Autodesk Inventor part; units mm, degrees
ref_plane "Work Plane1" through (0, 5, -20) normal (0, 1, 0) x (1, 0, 0)
ref_plane "YZ Plane" through (0, 0, 0) normal (1, 0, 0) x (0, 1, 0)
ref_plane "XZ Plane" through (0, 0, 0) normal (0, 1, 0) x (-1, 0, 0)
sketch "Sketch1" plane through (0, 0, 0) normal (1, 0, 0) x (0, 1, 0)
  line L0 (0, 0) -> (5, 0)
  line L1 (5, 0) -> (5, -40)
  line L2 (5, -40) -> (0, -40)
  line L3 (0, -40) -> (0, 0)
  line L4 (0, 0) -> (2.5, 0)
  line L5 (2.5, 0) -> (2.5, 16)
  line L6 (2.5, 16) -> (0, 16)
  line L7 (0, 16) -> (0, 0)
  line L8 (0, -40) -> (2.5, -40)
  line L9 (2.5, -40) -> (2.5, -54)
  line L10 (2.5, -54) -> (0, -54)
  line L11 (0, -54) -> (0, -40)
  line L12 (0, -54) -> (2.5, -54)
  line L13 (2.5, -54) -> (2.5, -61.5)
  line L14 (2.5, -61.5) -> (0, -61.5)
  line L15 (0, -61.5) -> (0, -54)
  line L16 (0, 16) -> (2, 16)
  line L17 (0, 14) -> (0, 16)
  line L18 (0, 19.99) -> (0, -68.5807)
  point P0 (2.5, -40)
  dimension "d0" = 5
  dimension "d1" = 40
  dimension "d2" = 2.5
  dimension "d3" = 16
  dimension "d4" = 2.5
  dimension "d5" = 14
  dimension "d6" = 2.5
  dimension "d7" = 7.5
revolve "Revolution1" add sketch "Sketch1" angle 360 about axis through (0, 0, 19.99) along (0, 0, -1)
sketch "Sketch4" plane through (0, 0, 0) normal (0, 0, 1) x (1, 0, 0)
  circle A0 centre (0, 0) radius 5 construction
  line L0 (0, 5) -> (2.5, 5)
  line L1 (2.5, 5) -> (-2.5, 5)
  line L2 (-2.5, 5) -> (-2.5, 3.5)
  line L3 (-2.5, 3.5) -> (2.5, 3.5)
  line L4 (2.5, 3.5) -> (2.5, 5)
  point P0 (0, 0)
  dimension "d25" = 2.5
  dimension "d26" = 5
  dimension "d27" = 1.5
extrude "Extrusion3" cut sketch "Sketch4" against normal blind 5.5
sketch "Sketch5" plane through (0, 0, -40) normal (0, 0, -1) x (-1, 0, 0)
  circle A0 centre (0, 0) radius 5 construction
  line L0 (0, 5) -> (2.5, 5)
  line L1 (-2.5, 4.3301) -> (-2.5, 3.5)
  line L2 (2.5, 5) -> (-2.5, 5)
  line L3 (-2.5, 5) -> (-2.5, 3.5)
  line L4 (-2.5, 3.5) -> (2.5, 3.5)
  line L5 (2.5, 3.5) -> (2.5, 5)
  point P0 (0, 0)
  dimension "d30" = 2.5
  dimension "d31" = 5
  dimension "d32" = 1.5
extrude "Extrusion4" cut sketch "Sketch5" against normal blind 5.5
ref_plane "Work Plane1" through (0, 5, -20) normal (0, 1, 0) x (1, 0, 0)
sketch "Sketch6" plane through (0, 5, -20) normal (0, 1, 0) x (1, 0, 0)
  line L0 (2.5, -14.5) -> (-2.5, -14.5)
  circle A0 centre (0, -14.5) radius 2.5
  line L1 (-2.5, 14.5) -> (2.5, 14.5)
  circle A1 centre (0, 14.5) radius 2.5
  point P0 (0, -20)
extrude "Extrusion5" cut sketch "Sketch6" against normal blind 1.5
fillet "Fillet2" radius 0.5 2 edges at (0, -2.5, 0) (0, -2.5, -40)
fillet "Fillet3" radius 0.25 6 edges at (0, 3.5, -8) (2.5, 3.5, -2.75) (-2.5, 3.5, -2.75) (0, 3.5, -32) (2.5, 3.5, -37.25) (-2.5, 3.5, -37.25)
properties part number "eje2" material "PBT Plastic"
Can you work these out from the model? Positions are in its coordinate system, mm. A direction names the side the tool comes from. Round coordinates to 2 decimals unless told otherwise and drop trailing zeros. Order: outer loops, then holes, each group sorted by start corner. A loop starts at its lowest first (then second) coordinate and runs counter-clockwise, first axis right, second up.
(1) If I drill on L1, parallel to Z at x = -3, y = 2.5; L2, parallel to Y at x = -0.5, z = -7.5; L3, parallel to X at y = 0.75, z = -21, over which ranges is the centre line in solid material (lowest first)?
Results are:
L1: z = -40 to 0
L2: y = -4.97 to 3.5
L3: x = -4.94 to 4.94
(2) If we section it at B-B (y = 0): Please give me the cut outline in (x, z), plus the area to 3 significant figures.
Results are:
outline: (-5, -40) - (-3, -40) arc R0.5 cw to (-2.5, -40.5) - (-2.5, -61.5) - (2.5, -61.5) - (2.5, -40.5) arc R0.5 cw to (3, -40) - (5, -40) - (5, 0) - (3, 0) arc R0.5 cw to (2.5, 0.5) - (2.5, 16) - (-2.5, 16) - (-2.5, 0.5) arc R0.5 cw to (-3, 0) - (-5, 0) - close
area: 588 mm2
(3) I'm going to push flat-ended pins straight in: pin 1 (3.5 mm diameter, centred on x = -0.5, z = -37.5, fed in from +Y); pin 2 (1.5 mm diameter, centred on y = 3.5, z = -24, fed in from -X); pin 3 (0.5 mm diameter, centred on y = 4, z = -37, fed in from +X). Where does each tip first touch, or does it pass through?
Results are:
pin 1: stops at y = 3.5
pin 2: stops at x = -4.18
pin 3: stops at x = 3.31
(4) If we section it at D-D (y = -3.75): Please give me the cut outline in (x, z).
Results are:
outline: (-3.31, -40) - (3.31, -40) - (3.31, 0) - (-3.31, 0) - close
(5) If we section it at C-C (z = -28.5): Please give me the cut outline in (x, y), plus the area to 3 significant figures.
Results are:
outline: circle Ø10 at (0, 0)
area: 78.5 mm2
(6) On a 3-axis mill with a long thin cutter (end or side, diameter ignored), from which of +Z, -Z, +X, -X, +Y, -Y can I reach the whole of each face in a straight line? I mean faces 1 (the face through (0, 3.5, -4)), 2 (the face through (0, 3.5, -36)), 3 (the face through (2.44, -0.54, 8.36)), 4 (the face through (-2.44, -0.54, -51.15)). Say none if no direction works.
Results are:
face 1: +Z, +Y
face 2: -Z, +Y
face 3: +Z
face 4: -Z
(7) If we section it at A-A (x = 0): Please give me the cut outline in (y, z).
Results are:
outline: (-5, -40) - (-3, -40) arc R0.5 cw to (-2.5, -40.5) - (-2.5, -61.5) - (2.5, -61.5) - (2.5, -40.5) arc R0.5 cw to (3, -40) - (3.5, -40) - (3.5, -32.25) arc R0.25 cw to (3.75, -32) - (5, -32) - (5, -8) - (3.75, -8) arc R0.25 cw to (3.5, -7.75) - (3.5, 0) - (3, 0) arc R0.5 cw to (2.5, 0.5) - (2.5, 16) - (-2.5, 16) - (-2.5, 0.5) arc R0.5 cw to (-3, 0) - (-5, 0) - close
